Autodesk Inventor part; units mm, degrees
ref_plane "YZ Plane" through (0, 0, 0) normal (1, 0, 0) x (0, 1, 0)
ref_plane "XZ Plane" through (0, 0, 0) normal (0, 1, 0) x (-1, 0, 0)
ref_plane "XY Plane" through (0, 0, 0) normal (0, 0, 1) x (1, 0, 0)
sketch "Sketch1" plane through (0, 0, 0) normal (0, 0, 1) x (1, 0, 0)
  arc A0 (-19.4827, -3.287) -> (-19.05, 0) centre (-31.75, 0) ccw
  line L0 (-19.4827, -3.287) -> (-58.7375, -149.7878)
  line L1 (-65.8876, 46.8376) -> (-65.8876, 21.4376)
  line L2 (-65.8876, 21.4376) -> (-71.4375, 21.4376)
  arc A1 (-19.05, 0) -> (-65.8876, 46.8376) centre (-65.8876, 0) ccw
  line L3 (-44.45, 34.1376) -> (-33.8192, 34.1376)
  line L4 (-44.45, 34.1376) -> (-37.3992, -46.4536)
  line L5 (-44.45, 34.1376) -> (0, 34.1376) construction
  line L6 (-37.3992, -46.4536) -> (-31.0492, -46.4536)
  line L7 (-71.4375, 21.4376) -> (-71.4375, 8.7376)
  line L8 (-71.4375, 8.7376) -> (-58.7375, 8.7376)
  line L9 (-58.7375, 8.7376) -> (-52.3875, 8.7376)
  line L10 (-52.3875, 8.7376) -> (-52.3875, -102.3907)
  line L11 (-71.4375, 8.7376) -> (-71.4375, -0.7874)
  line L12 (-71.4375, 8.7376) -> (-61.9125, 8.7376) construction
  line L13 (-71.4375, -0.7874) -> (-58.7375, -0.7874)
  line L14 (-58.7375, -0.7874) -> (-58.7375, -51.5874)
  line L15 (-58.7375, -51.5874) -> (-71.4375, -51.5874)
  line L16 (-71.4375, -0.7874) -> (-65.0875, -0.7874)
  line L17 (-65.0875, -0.7874) -> (-65.0875, -6.731)
  line L18 (-65.0875, -6.731) -> (-71.4375, -6.731)
  line L19 (-71.4375, 21.4376) -> (-71.4375, -0.7874)
  line L20 (-71.4375, -6.731) -> (-71.4375, -51.5874)
  line L21 (-58.7375, -51.5874) -> (-58.7375, -126.0892)
  line L22 (-58.7375, -51.5874) -> (0, -51.5874) construction
  line L23 (-46.0375, -102.3907) -> (-52.3875, -102.3907)
  line L24 (-65.0875, -51.5907) -> (-58.7375, -51.5907)
  line L25 (-58.7375, -149.7878) -> (-61.9125, -161.637)
  line L26 (-58.7375, -149.7878) -> (-34.203, -149.7878) construction
  line L27 (-65.0875, -161.637) -> (-61.9125, -161.637)
  line L28 (-58.7375, -126.0892) -> (-52.3875, -126.0892)
  line L29 (0, 34.1376) -> (0, 0)
  line L30 (-65.0875, -100.6892) -> (-65.0875, -161.637)
  line L31 (-58.7375, -51.5907) -> (-61.9125, -51.5907)
  line L32 (-65.0875, -100.6892) -> (-58.7375, -100.6892)
  dimension "d0" = 19.05
  dimension "d1" = 25.4
  dimension "d2" = 5.5499
  dimension "d3" = 65.8876
  dimension "d4" = 85
  dimension "d5" = 12.7
  dimension "d6" = 46.8376
  dimension "d7" = 12.7
  dimension "d8" = 44.45
  dimension "d9" = 6.35
  dimension "d10" = 105
  dimension "d11" = 12.7
  dimension "d12" = 12.7
  dimension "d13" = 6.35
  dimension "d14" = 9.525
  dimension "d15" = 50.8
  dimension "d16" = 12.7
  dimension "d17" = 6.35
  dimension "d18" = 5.9436
  dimension "d19" = 6.35
  dimension "d20" = 50.8
  dimension "d21" = 6.35
  dimension "d22" = 105
  dimension "d23" = 3.175
  dimension "d24" = 6.35
  dimension "d25" = 60.9478
  dimension "d26" = 3.175
  dimension "d27" = 6.35
revolve "Revolution1" add sketch "Sketch1" angle 360 about axis through (0, 34.1376, 0) along (0, -1, 0) contours L0 L25 L27 L30 L32 L21 L28
properties part number "Aluminum Skirt" material "Aluminum 6061"
Geometry: final body of the model. Coordinates: model frame, mm. A direction names the side the tool comes from. Coordinates: 2 decimals unless noted, no trailing zeros. Write each loop counter-clockwise with the first axis right and the second up, starting at its lowest first coordinate (ties: lowest second). Pieces come first, ordered by that corner, then holes. Notation, with made-up numbers: M 85.25,25.5 L 112.25,25.5 A31 ccw 112.25,52.5 Z; hole C -17.5,65.25 d4. An arc over 180 degrees is marked long. Use CSV: the item, a comma, the result in double quotes. Start each with the question number.
1. Cut plane A-A on z = 0. Return the cut outline in (x, y), plus the area to 3 significant figures.
2. Cut plane B-B on x = 0. Return the cut outline in (y, z).
3. Ray query, probe 1 along X at (y, z) = (-112, 0); probe 2 along X at (y, z) = (-148, -50); probe 3 along Z at (x, y) = (27.5, -112). Return the intervals inside material, ascending.
4. Reachability of faces 1 (the face through (46.612, -113.567, 35.741)), 2 (the face through (-58, -161.637, 24)) from +Z, -Z, +X, -X, +Y, -Y: full face, straight path, thin tool, end or side. Return the list, or none.
5. Mould query, pull axis Z, two halves, no side actions, for faces 3 (the face through (9.9, -100.689, -58.2)), 4 (the face through (51.651, -131.59, 39.605)), 5 (the face through (52.5, -126.089, 4.1)). Classes: pulls with the +Z half, pulls with the -Z half, needs draft (parallel to the pull), parting line crosses it, or undercut.
6. First-contact query: P1, Ø10, axis at y = -110, z = -16.5, coming from the +X side; P2, Ø4, axis at x = -29, y = -133.5, coming from the +Z side; P3, Ø10, axis at x = -14.5, y = -123, coming from the -Z side. Flat tips, straight axial feed; report the tip coordinate or a pass-through.
Entries:
1,outline,"M -65.09,-161.64 L -61.91,-161.64 L -58.74,-149.79 L -52.39,-126.09 L -58.74,-126.09 L -58.74,-100.69 L -65.09,-100.69 Z; M 52.39,-126.09 L 58.74,-149.79 L 61.91,-161.64 L 65.09,-161.64 L 65.09,-100.69 L 58.74,-100.69 L 58.74,-126.09 Z"
1,area,"887 mm²"
2,outline,"M -161.64,-65.09 L -100.69,-65.09 L -100.69,-58.74 L -126.09,-58.74 L -126.09,-52.39 L -149.79,-58.74 L -161.64,-61.91 Z; M -161.64,61.91 L -149.79,58.74 L -126.09,52.39 L -126.09,58.74 L -100.69,58.74 L -100.69,65.09 L -161.64,65.09 Z"
3,probe 1,"-65.09 to -58.74, 58.74 to 65.09"
3,probe 2,"-41.67 to -29.9, 29.9 to 41.67"
3,probe 3,"-58.99 to -51.9, 51.9 to 58.99"
4,face 1,"+Y"
4,face 2,"+Z, -Z, +X, -X, -Y"
5,face 3,"needs draft"
5,face 4,"parting line crosses it"
5,face 5,"undercut"
6,P1,"x = 64.06"
6,P2,"z = 59.22"
6,P3,"z = -64.39"
